The model under review builds one solid part; all positions refer to its coordinate system, in mm. Give positions to 0.01 mm unless a question says otherwise; leave off trailing zeros. Loops run counter-clockwise (first coordinate to the right, second up) from the corner with the lowest first, then second, coordinate; pieces in that order, holes last. Notation, with made-up numbers: (14.25, 51) - (25.25, 51) arc R21 ccw to (25.25, 89) - close; hole circle Ø8 at (-16.5, -20.75). An arc over 180 degrees is marked (long way). Return JSON: item names as keys, results as strings. Group by question number.
from build123d import *

# Parameters (mm, degrees)
SKETCH1_W           = 59
SKETCH1_H           = 50
SKETCH1_R           = 9.55
BOSS_EXTRUDE1_DEPTH = 4
CHAMFER1_SIZE       = 4


with BuildPart() as part:
    # Sketch1 → Boss-Extrude1 (new body)
    with BuildSketch(Plane(origin=(0, 0, 0), x_dir=(1, 0, 0), z_dir=(0, 1, 0))):
        with Locations((29.5, 25)):
            Rectangle(SKETCH1_W, SKETCH1_H)
        with Locations(Location((29.5, 25, 0), (0, 0, 270))):
            Circle(SKETCH1_R, mode=Mode.SUBTRACT)
    extrude(amount=BOSS_EXTRUDE1_DEPTH)

    # Chamfer1
    chamfer1_edges = [part.edges().sort_by_distance(p)[0] for p in [
        (29.5, 4, -50),
        (29.5, 4, 0),
    ]]
    chamfer(chamfer1_edges, length=CHAMFER1_SIZE - 0.0001)  # a hair under: the kernel refuses the full size


solid = part.part
Item 1: Take a section at B-B (z = -25). State the section outline as (x, y) points, then the cut area to 3 significant figures.
Item 2: Take a section at D-D (y = 2.8). State the section outline as (x, z) points, then the cut area to 3 significant figures.
Item 3: For P1, Ø1.5, axis at x = 12, y = 1, coming from the -Z side, flat-tipped, find the tip position at first contact; note if it passes through.
Item 4: For L1, parallel to X at y = 2.4, z = -25; L2, parallel to Z at x = 24, y = 1.35; L3, parallel to X at y = 0.65, z = -32, list the stretches that pass through material, from the lowest coordinate up. Write a range as from..to.
Item 5: Mouldability with a two-part tool opening along Z and no side actions: class faces 1 (the face through (29, 2, -2)), 2 (the face through (21.03, 1.97, -20.59)), 3 (the face through (29, 4, -35)) as +Z half, -Z half, draft (parallel to the pull), parting line (faces both ways), or undercut.
Check sheet entries:
{
 "1": {"outline": "(0, 0) - (19.95, 0) - (19.95, 4) - (0, 4) - close; (39.05, 0) - (59, 0) - (59, 4) - (39.05, 4) - close", "area": "160 mm^2"},
 "2": {"outline": "(0, -47.2) - (59, -47.2) - (59, -2.8) - (0, -2.8) - close; hole circle Ø19.1 at (29.5, -25)", "area": "2,330 mm^2"},
 "3": {"P1": "stops at z = -49.75"},
 "4": {"L1": "x = 0..19.95, 39.05..59", "L2": "z = -48.65..-32.81, -17.19..-1.35", "L3": "x = 0..23, 36..59"},
 "5": {"face 1": "+Z half", "face 2": "undercut", "face 3": "draft"}
}
